Here's the drawing with two shaded views (mm, measured from the low corner). I have some questions. A direction names the side the tool comes from. Round coordinates to 2 decimals unless told otherwise and drop trailing zeros. Loops run counter-clockwise (first coordinate to the right, second up) from the corner with the lowest first, then second, coordinate; pieces in that order, holes last. Notation, with made-up numbers: M 54.5,26 L 65.5,26 A36 ccw 65.5,62 Z; hole C 71,42 d5. An arc over 180 degrees is marked long. One line per item, written item: value. Start each with the question number.
Q1. Which directions (+Z, -Z, +X, -X, +Y, -Y) give clear straight access to the entire face, cutting with the end or side of a thin tool? Please do the marked faces 4, 5 and 6.
Q2. I'm going to push flat-ended pins straight in: pin 1 Ø6 at (x, y) = (6, 11) entering from +Z (1 decimal); pin 2 Ø5 at (x, z) = (12.5, 16.5) entering from +Y (1 decimal); pin 3 Ø11.5 at (x, z) = (15, 12.5) entering from +Y. Where does each tip first touch, or does it pass through?
Q3. Thinking about a two-plate mould opening in X: for the marked faces 1, 2 and 3, which applies, released by +X, released by -X, zero draft, split by the parting line, or undercut?
Q4. Imagine slicing it at C-C (y = 21.5). Please give me the cut outline in (x, z).
Q5. Imagine slicing it at B-B (z = 12.5). Please give me the cut outline in (x, y), then the cut area to 3 significant figures.
Q6. Imagine slicing it at D-D (x = 8). Please give me the cut outline in (y, z) (1 decimal).
Q7. Please list where these lines run through material, in increasing order: line 1 along X through (y, z) = (9.9, 1.65); line 2 along X through (y, z) = (19.25, 2.75); line 3 along Y through (x, z) = (26, 15.5).
Q8. Imagine slicing it at A-A (x = 15). Please give me the cut outline in (y, z).
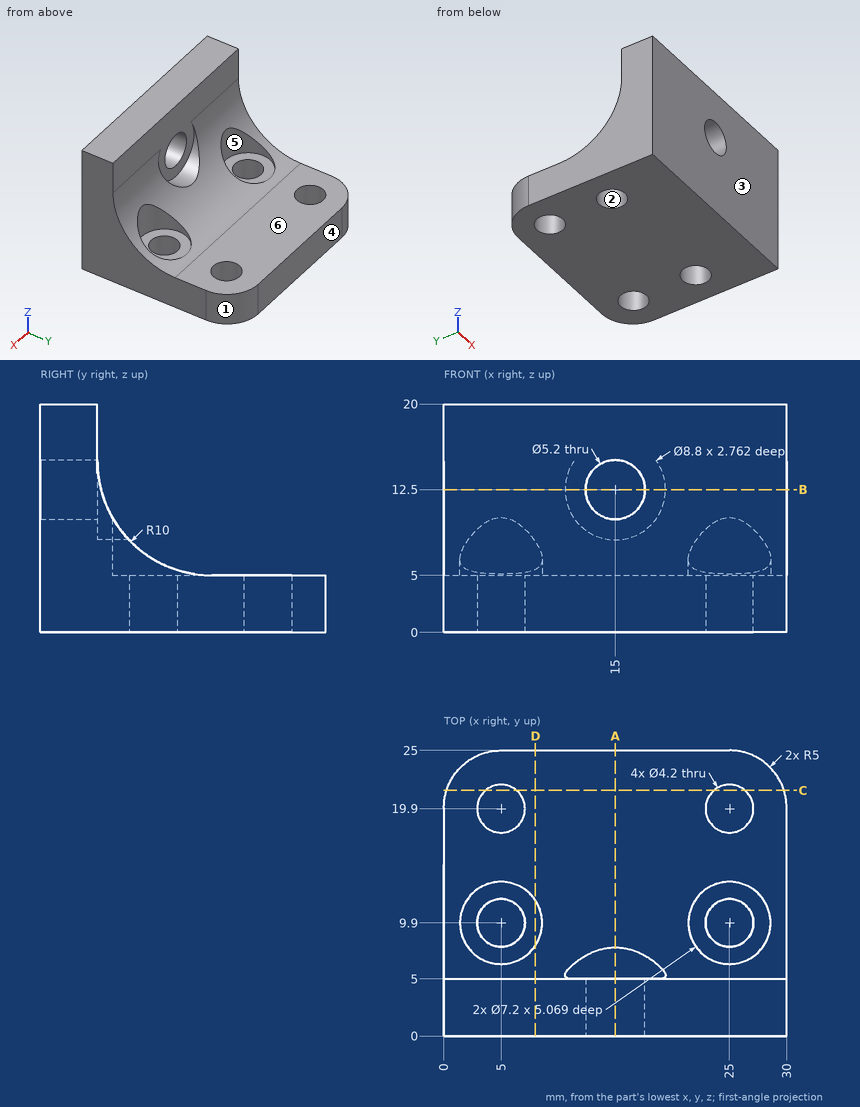
Report:
1. face 4: +Z, -Z, +X, -X, +Y
1. face 5: +Z
1. face 6: +Z, +X, -X, +Y
2. pin 1: stops at z = 6.7
2. pin 2: stops at y = 5
2. pin 3: stops at y = 9.35
3. face 1: released by +X
3. face 2: undercut
3. face 3: zero draft
4. outline: M 0.23,0 L 3.64,0 L 3.64,5 L 0.23,5 Z; M 6.36,0 L 23.64,0 L 23.64,5 L 6.36,5 Z; M 26.36,0 L 29.77,0 L 29.77,5 L 26.36,5 Z
5. outline: M 0,0 L 12.4,0 L 12.4,5 L 10.6,5 L 10.6,5.32 L 0,5.32 Z; M 17.6,0 L 30,0 L 30,5.32 L 19.4,5.32 L 19.4,5 L 17.6,5 Z
5. area: 131 mm²
6. outline: M 0,0 L 25,0 L 25,5 L 15,5 A10 cw 11.9,5.5 L 11.9,5 L 7.9,5 L 7.9,7.9 A10 cw 5,15 L 5,20 L 0,20 Z
7. line 1: x = 0 to 2.9, 7.1 to 22.9, 27.1 to 30
7. line 2: x = 0 to 3, 7 to 23, 27 to 30
7. line 3: y = 0 to 5
8. outline: M 0,0 L 25,0 L 25,5 L 15,5 A10 cw 7.76,8.1 L 5,8.1 L 5,9.9 L 0,9.9 Z; M 0,15.1 L 5,15.1 L 5,20 L 0,20 Z
